```python
from build123d import *

# Parameters (mm, degrees)
SKETCH_1_R                  = 18
EXTRUDE_1_DEPTH             = 11
HOLE_WIZARD_M8_1_AT_2_COUNT = 2
HOLE_WIZARD_M8_1_AT_2_PITCH = 90
HOLE_WIZARD_M6_1_D          = 5
HOLE_WIZARD_M6_1_DEPTH      = 15
HOLE_WIZARD_M6_1_TIP        = 1.502151548


with BuildPart() as part:
    # 草图1 → 拉伸1 (new, symmetric)
    with BuildSketch(Plane.XY):
        Polygon((35, 18), (55, 18), (55, 0), (-55, 0), (-55, 18), (-35, 18), (-35, 68), (-30, 73), (30, 73), (35, 68), align=None)
        with Locations((0, 40)):
            Circle(SKETCH_1_R, mode=Mode.SUBTRACT)
    extrude(amount=EXTRUDE_1_DEPTH, both=True)

    # 草图2 → M8 六角凹头螺钉的柱形沉头孔1 (revolve, cut)
    with BuildSketch(Plane(origin=(-45, 18, 0), x_dir=(0, 0, 1), z_dir=(1, 0, 0))):
        Polygon((0, 0), (0, 18), (4.5, 18), (4.5, 8), (7.5, 8), (7.5, 0.025), (7.525, 0), align=None)
    hole_wizard_m8_1 = revolve(axis=Axis((-45, 24.35, 0), (0, -1, 0)), mode=Mode.SUBTRACT)

    # M8 六角凹头螺钉的柱形沉头孔1 at 2: M8 六角凹头螺钉的柱形沉头孔1 ×2
    with Locations(*[(i * HOLE_WIZARD_M8_1_AT_2_PITCH, 0, 0) for i in range(1, HOLE_WIZARD_M8_1_AT_2_COUNT)]):
        add(hole_wizard_m8_1, mode=Mode.SUBTRACT)

    # M6 螺纹孔1
    with Locations(Plane(origin=(0, 0, -11), x_dir=(-1, 0, 0), z_dir=(0, 0, -1))):
        with Locations((16.615900688, 25.382990642), (-16.618118028, 25.382990642), (-23.50110867, 42), (-16.618118028, 58.617009358), (16.615900688, 58.617009358), (23.49889133, 42)):
            Hole(HOLE_WIZARD_M6_1_D / 2, depth=HOLE_WIZARD_M6_1_DEPTH)
            with Locations((0, 0, -(HOLE_WIZARD_M6_1_DEPTH + HOLE_WIZARD_M6_1_TIP / 2))):  # 118° drill point
                Cone(0, HOLE_WIZARD_M6_1_D / 2, HOLE_WIZARD_M6_1_TIP, mode=Mode.SUBTRACT)


solid = part.part
```
Here's how the part is built. I have some questions about the finished solid (model axes, mm). A direction names the side the tool comes from. Give positions to 0.01 mm unless a question says otherwise; leave off trailing zeros. Write each loop counter-clockwise with the first axis right and the second up, starting at its lowest first coordinate (ties: lowest second). Pieces come first, ordered by that corner, then holes. Notation, with made-up numbers: M 21.25,82 L 26.25,82 A17 cw 26.25,100 Z; hole C 65,14.25 d3. An arc over 180 degrees is marked long. Put each result on its own line as item: value. Start each with the question number.
Item 1: Will these pins go through, and if not, where does the flat tip stop? pin 1 (8 mm diameter, centred on x = -16.62, y = 25.38, fed in from -Z); pin 2 (1.5 mm diameter, centred on y = 25, z = 6, fed in from -X); pin 3 (4 mm diameter, centred on x = -16.62, y = 58.62, fed in from -Z); pin 4 (7.5 mm diameter, centred on x = 44.5, z = -2, fed in from +Y).
Item 2: On a 3-axis mill with a long thin cutter (end or side, diameter ignored), from which of +Z, -Z, +X, -X, +Y, -Y can I reach the whole of each face in a straight line? I mean faces 1 (the cylindrical face through (22.96, 39.56, -3.39)), 2 (the flat face through (45, 10, -5)), 3 (the flat face through (-47.4, 18, 7.5)). Say none if no direction works.
Item 3: If we section it at A-A, the plane x = 0: Write out the boundary of the cut face in (y, z), then the cut area to 3 significant figures.
Item 4: Thinking about a two-plate mould opening in X: for faces 4 (the flat face through (-55, 9, 0)), 5 (the flat face through (1, 0, 0)), 6 (the cylindrical face through (-2.343, 57.847, -0.154)), 7 (the cylindrical face through (-24.04, 39.56, -3.39)), which applies, +X half, -X half, draft (parallel to the pull), parting line (faces both ways), or undercut?
Item 5: If we section it at B-B, the plane x = -45: Write out the boundary of the cut face in (y, z) (3 decimals), then the cut area to 3 significant figures.
Item 6: If we section it at D-D, the plane y = 65: Write out the boundary of the cut face in (x, z), then the cut area to 3 significant figures.
Item 7: If we section it at C-C, the plane y = 49: Write out the boundary of the cut face in (x, z), then the cut area to 3 significant figures.
Item 8: I need wall thicknesses on L1, parallel to X at y = 9, z = 0; L2, parallel to Z at x = -45, y = 4; L3, parallel to X at y = 42.5, z = -3.25. Which ranges of each line are inside material? Lowest first, please. Write a range as from..to.
Values:
1. pin 1: z = -11
1. pin 2: x = -35
1. pin 3: z = 4.3
1. pin 4: y = 10
2. face 1: -Z
2. face 2: +Y
2. face 3: +Z, -Z, -X, +Y
3. outline: M 0,-11 L 22,-11 L 22,11 L 0,11 Z; M 58,-11 L 73,-11 L 73,11 L 58,11 Z
3. area: 814 mm²
4. face 4: -X half
4. face 5: draft
4. face 6: undercut
4. face 7: undercut
5. outline: M 0,-11 L 18,-11 L 18,-7.525 L 17.975,-7.5 L 10,-7.5 L 10,-4.5 L 0,-4.5 Z; M 0,4.5 L 10,4.5 L 10,7.5 L 17.975,7.5 L 18,7.525 L 18,11 L 0,11 Z
5. area: 186 mm²
6. outline: M -35,-11 L 35,-11 L 35,11 L -35,11 Z
6. area: 1,540 mm²
7. outline: M -35,-11 L -15.59,-11 L -15.59,11 L -35,11 Z; M 15.59,-11 L 35,-11 L 35,11 L 15.59,11 Z
7. area: 854 mm²
8. L1: -55..-49.5, -40.5..40.5, 49.5..55
8. L2: -11..-4.5, 4.5..11
8. L3: -35..-25.95, -21.05..-17.83, 17.83..21.05, 25.95..35
